Part print with two shaded views. Sizes in mm from the minimum x, y, z corner. A direction names the side the tool comes from. Coordinates: 2 decimals unless noted, no trailing zeros. Order: outer loops, then holes, each group sorted by start corner. A loop starts at its lowest first (then second) coordinate and runs counter-clockwise, first axis right, second up. Notation, with made-up numbers: (85, 69.5) - (98, 69.5) arc R27 cw to (98, 105.5) - close; hole circle Ø9 at (14, 31.25). An arc over 180 degrees is marked (long way). Return JSON: item names as keys, results as strings.
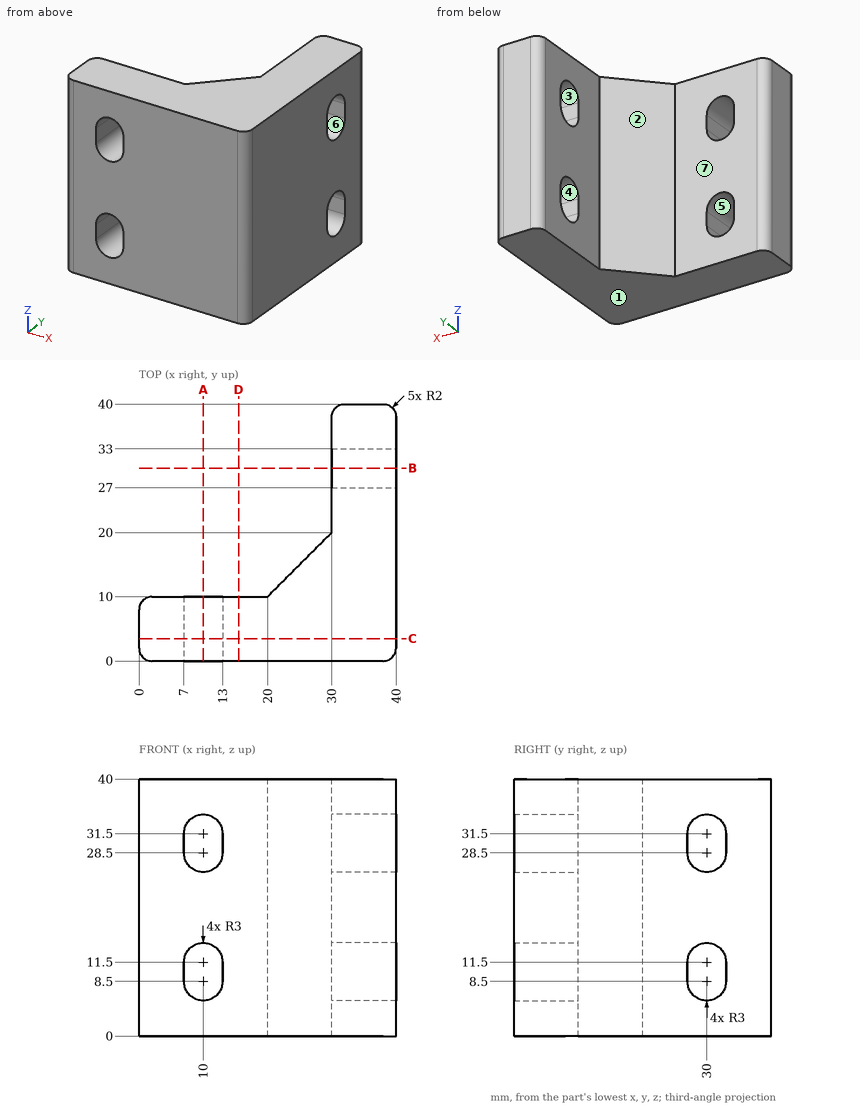
Item 1: Drop flat-ended pins along their axis: P1, Ø10, axis at y = 19, z = 12.5, coming from the -X side; P2, Ø12, axis at x = 13, y = 18.5, coming from the +Z side; P3, Ø20, axis at y = 32.5, z = 20, coming from the -X side; P4, Ø12, axis at y = 18.5, z = 20.5, coming from the -X side. Give the stop position or say it passes through.
Findings below:
{"P1": "stops at x = 24", "P2": "passes through", "P3": "stops at x = 30", "P4": "stops at x = 22.5"}
Item 2: Band-saw the part on D-D, the plane x = 15.5. List the corners of the cut face in (y, z), then the cut area to 3 significant figures.
Findings below:
{"outline": "(0, 0) - (10, 0) - (10, 40) - (0, 40) - close", "area": "400 mm²"}
Item 3: Band-saw the part on C-C, the plane y = 3.5. List the corners of the cut face in (x, z).
Findings below:
{"outline": "(0, 0) - (40, 0) - (40, 40) - (0, 40) - close; hole (7, 8.5) arc R3 ccw to (13, 8.5) - (13, 11.5) arc R3 ccw to (7, 11.5) - close; hole (7, 28.5) arc R3 ccw to (13, 28.5) - (13, 31.5) arc R3 ccw to (7, 31.5) - close"}
Item 4: Wall check: L1, parallel to Y at x = 24.5, z = 20; L2, parallel to X at y = 20.5, z = 27; L3, parallel to Y at x = 16, z = 12. Give the ranges that are in metal, low to high. Write a range as [from, to].
Findings below:
{"L1": "y = [0, 14.5]", "L2": "x = [30, 40]", "L3": "y = [0, 10]"}
Item 5: Band-saw the part on B-B, the plane y = 30. List the corners of the cut face in (x, z).
Findings below:
{"outline": "(30, 0) - (40, 0) - (40, 5.5) - (30, 5.5) - close; (30, 14.5) - (40, 14.5) - (40, 25.5) - (30, 25.5) - close; (30, 34.5) - (40, 34.5) - (40, 40) - (30, 40) - close"}
Item 6: Mould opens along Y. For the marked faces 1, 2, 3 and 4 say: released by +Y, released by -Y, zero draft, split by the parting line, or undercut.
Findings below:
{"face 1": "zero draft", "face 2": "released by +Y", "face 3": "undercut", "face 4": "undercut"}
Item 7: Which spindle directions (+Z, -Z, +X, -X, +Y, -Y) get a long thin tool onto all of the face, cutting with end or side? Do the marked faces 5, 6 and 7. Say none if no direction does.
Findings below:
{"face 5": "+Y, -Y", "face 6": "+X, -X", "face 7": "+Z, -Z, -X, +Y"}
Item 8: Band-saw the part on A-A, the plane x = 10. List the corners of the cut face in (y, z).
Findings below:
{"outline": "(0, 0) - (10, 0) - (10, 5.5) - (0, 5.5) - close; (0, 14.5) - (10, 14.5) - (10, 25.5) - (0, 25.5) - close; (0, 34.5) - (10, 34.5) - (10, 40) - (0, 40) - close"}
